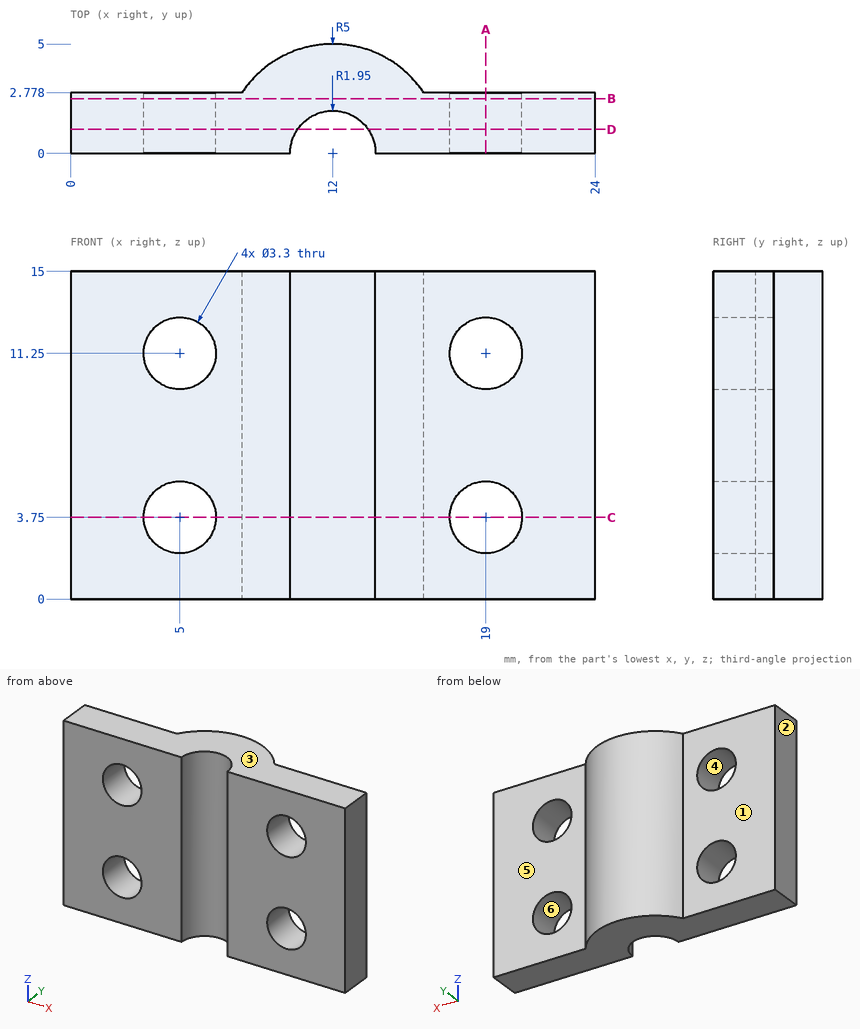
The drawing under review shows one solid part. Ordinate dimensions are in mm from its lowest x, y, z. A direction names the side the tool comes from. Round coordinates to 2 decimals unless told otherwise and drop trailing zeros. Write each loop counter-clockwise with the first axis right and the second up, starting at its lowest first coordinate (ties: lowest second). Pieces come first, ordered by that corner, then holes.
(1) We need section B-B on y = 2.5. Give the boundary of the cut face in (x, z), and give its area (3 significant figures).
(2) Mouldability with a two-part tool opening along Z and no side actions: class the marked faces 3, 4, 5 and 6 as +Z half, -Z half, draft (parallel to the pull), parting line (faces both ways), or undercut.
(3) Machinability: for the marked faces 1 and 2, which of the approach directions +Z, -Z, +X, -X, +Y, -Y give a long, thin tool a straight path to every point of the face, cutting with its end or side? Answer none if there is none.
(4) Wall thickness on L1, parallel to X at y = 2.15, z = 11.25; L2, parallel to Z at x = 19.25, y = 1.85; L3, parallel to Z at x = 17.5, y = 1.85 (1 decimal): over which ranges is each line inside the solid? List them lowest first.
(5) Insertion check: pin 1 (4.5 mm diameter, centred on x = 19, z = 3.75, fed in from -Y); pin 2 (2.5 mm diameter, centred on x = 3.5, z = 7.5, fed in from +Y); pin 3 (2.5 mm diameter, centred on x = 5, z = 11.25, fed in from -Y); pin 4 (2 mm diameter, centred on x = 14.5, z = 7.5, fed in from +Y). Each pin has a flat end and moves straight along its axis. Give the tip position at first contact, or say it passes through.
(6) We need section D-D on y = 1.1. Give the boundary of the cut face in (x, z).
(7) We need section A-A on x = 19. Give the boundary of the cut face in (y, z).
(8) We need section C-C on z = 3.75. Give the boundary of the cut face in (x, y).
Findings below:
1. outline: (0, 0) - (24, 0) - (24, 15) - (0, 15) - close; hole circle Ø3.3 at (5, 3.75); hole circle Ø3.3 at (5, 11.25); hole circle Ø3.3 at (19, 3.75); hole circle Ø3.3 at (19, 11.25)
1. area: 326 mm2
2. face 3: +Z half
2. face 4: undercut
2. face 5: draft
2. face 6: undercut
3. face 1: +Z, -Z, -X, +Y
3. face 2: +Z, -Z, -X, +Y, -Y
4. L1: x = 0 to 3.35, 6.65 to 17.35, 20.65 to 24
4. L2: z = 0 to 2.12, 5.38 to 9.62, 12.88 to 15
4. L3: z = 0 to 3.1, 4.4 to 10.6, 11.9 to 15
5. pin 1: stops at y = 0
5. pin 2: stops at y = 2.78
5. pin 3: passes through
5. pin 4: stops at y = 4.77
6. outline: (0, 0) - (10.39, 0) - (10.39, 15) - (0, 15) - close; (13.61, 0) - (24, 0) - (24, 15) - (13.61, 15) - close; hole circle Ø3.3 at (5, 3.75); hole circle Ø3.3 at (5, 11.25); hole circle Ø3.3 at (19, 3.75); hole circle Ø3.3 at (19, 11.25)
7. outline: (0, 0) - (2.78, 0) - (2.78, 2.1) - (0, 2.1) - close; (0, 5.4) - (2.78, 5.4) - (2.78, 9.6) - (0, 9.6) - close; (0, 12.9) - (2.78, 12.9) - (2.78, 15) - (0, 15) - close
8. outline: (0, 0) - (3.35, 0) - (3.35, 2.78) - (0, 2.78) - close; (6.65, 0) - (10.05, 0) arc R1.95 cw to (13.95, 0) - (17.35, 0) - (17.35, 2.78) - (16.16, 2.78) arc R5 ccw to (7.84, 2.78) - (6.65, 2.78) - close; (20.65, 0) - (24, 0) - (24, 2.78) - (20.65, 2.78) - close
